from build123d import *

# Parameters (mm, degrees)
F0_W     = 28
F0_H     = 15.127502
F0_R     = 4.75
F1_DEPTH = 15
F2_R     = 2.6
F3_DEPTH = 25
F2_R_2   = 3.5
F4_DEPTH = 4


with BuildPart() as f1:
    # F0 (on Top) → F1 (new body)
    with BuildSketch(Plane.XY):
        Rectangle(F0_W, F0_H)
        Circle(F0_R, mode=Mode.SUBTRACT)
    extrude(amount=-F1_DEPTH)

    # F2 (on face) → F3 (cut)
    with BuildSketch(Plane.XZ.offset(7.563751)):
        with Locations((-8, -7.5)):
            Circle(F2_R)
        with Locations((8, -7.5)):
            Circle(F2_R)
    extrude(amount=-F3_DEPTH, mode=Mode.SUBTRACT)

    # F2 (on face) → F4 (cut)
    with BuildSketch(Plane.XZ.offset(7.563751)):
        with Locations((-8, -7.5)):
            Circle(F2_R_2)
        with Locations((-8, -7.5)):
            Circle(F2_R, mode=Mode.SUBTRACT)
        with Locations((8, -7.5)):
            Circle(F2_R_2)
        with Locations((8, -7.5)):
            Circle(F2_R, mode=Mode.SUBTRACT)
    extrude(amount=-F4_DEPTH, mode=Mode.SUBTRACT)


solid = f1.part
Design review of the part built by this model. Coordinates are the model's own, in mm. A direction names the side the tool comes from. Round coordinates to 2 decimals unless told otherwise and drop trailing zeros. Order: outer loops, then holes, each group sorted by start corner. A loop starts at its lowest first (then second) coordinate and runs counter-clockwise, first axis right, second up.
1) Machinability: for faces 1 (the cylindrical face through (10.48, 1.92, -6.72)), 2 (the flat face through (-11, -3.564, -8)), which of the approach directions +Z, -Z, +X, -X, +Y, -Y give a long, thin tool a straight path to every point of the face, cutting with its end or side? Answer none if there is none.
The answers:
face 1: +Y, -Y
face 2: -Y
2) Draft analysis for pull direction Z (two halves, no side actions). For faces 3 (the flat face through (0, 5, 0)), 4 (the cylindrical face through (4.503, -5.592, -7.346)), 5 (the flat face through (-14, 0, -7)), 6 (the flat face through (0, 5, -15)), state which applies: released by +Z, released by -Z, zero draft, split by the parting line, or undercut.
The answers:
face 3: released by +Z
face 4: undercut
face 5: zero draft
face 6: released by -Z
3) Clearance check with a flat-ended pin moving along its axis: pin 1 Ø3.5 at (x, z) = (-7.5, -6) entering from -Y. State where the tip first meets the part, or that it passes through.
The answers:
pin 1: stops at y = -3.56
4) Consider section C-C (y = -3). State the section outline as (x, z) points.
The answers:
outline: (-14, -15) - (-3.68, -15) - (-3.68, 0) - (-14, 0) - close; (3.68, -15) - (14, -15) - (14, 0) - (3.68, 0) - close; hole circle Ø5.2 at (-8, -7.5); hole circle Ø5.2 at (8, -7.5)
5) For L1, parallel to Z at x = 8, y = -1.5; L2, parallel to Y at x = 0, z = -6; L3, parallel to X at y = -5.25, z = -8, list the stretches that pass through material, from the lowest coordinate up.
The answers:
L1: z = -15 to -10.1, -4.9 to 0
L2: y = -7.56 to -4.75, 4.75 to 7.56
L3: x = -14 to -11.46, -4.54 to 4.54, 11.46 to 14
6) Consider section B-B (x = 0). State the section outline as (y, z) points.
The answers:
outline: (-7.56, -15) - (-4.75, -15) - (-4.75, 0) - (-7.56, 0) - close; (4.75, -15) - (7.56, -15) - (7.56, 0) - (4.75, 0) - close
7) Consider section D-D (z = -13). State the section outline as (x, y) points, plus the area to 3 significant figures.
The answers:
outline: (-14, -7.56) - (14, -7.56) - (14, 7.56) - (-14, 7.56) - close; hole circle Ø9.5 at (0, 0)
area: 353 mm2
8) Consider section A-A (z = -7.5). State the section outline as (x, y) points.
The answers:
outline: (-14, -7.56) - (-11.5, -7.56) - (-11.5, -3.56) - (-10.6, -3.56) - (-10.6, 7.56) - (-14, 7.56) - close; (-5.4, -3.56) - (-4.5, -3.56) - (-4.5, -7.56) - (4.5, -7.56) - (4.5, -3.56) - (5.4, -3.56) - (5.4, 7.56) - (-5.4, 7.56) - close; (10.6, -3.56) - (11.5, -3.56) - (11.5, -7.56) - (14, -7.56) - (14, 7.56) - (10.6, 7.56) - close; hole circle Ø9.5 at (0, 0)
